Check sheet for the modelled part. Datum: model origin and axes. Units: mm. Face numbers are marked on the shaded views. A direction names the side the tool comes from. Round coordinates to 2 decimals unless told otherwise and drop trailing zeros. Loops run counter-clockwise (first coordinate to the right, second up) from the corner with the lowest first, then second, coordinate; pieces in that order, holes last. Notation, with made-up numbers: (22, -25) -> (79, -25) arc R16 cw to (79, -2) -> close; hole circle Ø7 at (31, 89). An arc over 180 degrees is marked (long way). One line per question, with ' | ' between items.
```python
from build123d import *

# Parameters (mm, degrees)
F0_W     = 50.8
F0_H     = 101.6
F0_W_2   = 101.6
F0_H_2   = 50.8
F1_DEPTH = 38.1
F2_W     = 30.8
F2_H     = 10
F2_W_2   = 10
F2_H_2   = 30.8
F2_W_3   = 30
F2_H_3   = 30
F3_DEPTH = 20
F4_SIZE  = 3
F5_SIZE  = 5


with BuildPart() as f1:
    # F0 (on Top) → F1 (new body)
    with BuildSketch(Plane.XY):
        with BuildLine():
            Line((0, 47.625), (0, 0))
            Line((0, 0), (50.8, 0))
            Line((50.8, 0), (50.8, 50.8))
            Line((50.8, 50.8), (3.175, 50.8))
            ThreePointArc((3.175, 50.8), (2.245064, 48.554936), (0, 47.625))
        make_face()
        with Locations((25.4, -50.8)):
            Rectangle(F0_W, F0_H)
        with Locations((101.6, 25.4)):
            Rectangle(F0_W_2, F0_H_2)
    extrude(amount=F1_DEPTH)

    # F2 (on face) → F3 (cut)
    with BuildSketch(Plane.XY.offset(38.1)):
        with Locations((25.4, -86.6)):
            Rectangle(F2_W, F2_H)
        with Locations((25.4, -61.6)):
            Rectangle(F2_W, F2_H)
        with Locations((25.4, -36.6)):
            Rectangle(F2_W, F2_H)
        with Locations((25.4, -11.6)):
            Rectangle(F2_W, F2_H)
        with Locations((137.4, 25.4)):
            Rectangle(F2_W_2, F2_H_2)
        with Locations((112.4, 25.4)):
            Rectangle(F2_W_2, F2_H_2)
        with Locations((87.4, 25.4)):
            Rectangle(F2_W_2, F2_H_2)
        with Locations((62.4, 25.4)):
            Rectangle(F2_W_2, F2_H_2)
        with Locations((25, 25.8)):
            Rectangle(F2_W_3, F2_H_3)
    extrude(amount=-F3_DEPTH, mode=Mode.SUBTRACT)

    # F4
    f4_edges = [f1.edges().sort_by_distance(p)[0] for p in [
        (10, -6.6, 28.1),
        (10, 40.8, 28.1),
        (10, -31.6, 28.1),
        (10, -56.6, 28.1),
        (10, -81.6, 28.1),
        (10, -91.6, 28.1),
        (40.8, -81.6, 28.1),
        (40.8, -91.6, 28.1),
        (40.8, -66.6, 28.1),
        (40.8, -56.6, 28.1),
        (10, -66.6, 28.1),
        (10, -41.6, 28.1),
        (40.8, -31.6, 28.1),
        (40.8, -41.6, 28.1),
        (10, -16.6, 28.1),
        (40.8, -16.6, 28.1),
        (40.8, -6.6, 28.1),
        (10, 10.8, 28.1),
        (40, 40.8, 28.1),
        (40, 10.8, 28.1),
        (57.4, 40.8, 28.1),
        (57.4, 10, 28.1),
        (67.4, 10, 28.1),
        (67.4, 40.8, 28.1),
        (82.4, 40.8, 28.1),
        (82.4, 10, 28.1),
        (92.4, 40.8, 28.1),
        (92.4, 10, 28.1),
        (107.4, 10, 28.1),
        (117.4, 10, 28.1),
        (117.4, 40.8, 28.1),
        (107.4, 40.8, 28.1),
        (132.4, 10, 28.1),
        (142.4, 10, 28.1),
        (142.4, 40.8, 28.1),
        (132.4, 40.8, 28.1),
    ]]
    chamfer(f4_edges, length=F4_SIZE)

    # F5
    f5_edges = [f1.edges().sort_by_distance(p)[0] for p in [
        (0, -101.6, 19.05),
        (50.8, -101.6, 19.05),
        (152.4, 0, 19.05),
        (152.4, 50.8, 19.05),
    ]]
    chamfer(f5_edges, length=F5_SIZE)


solid = f1.part
```
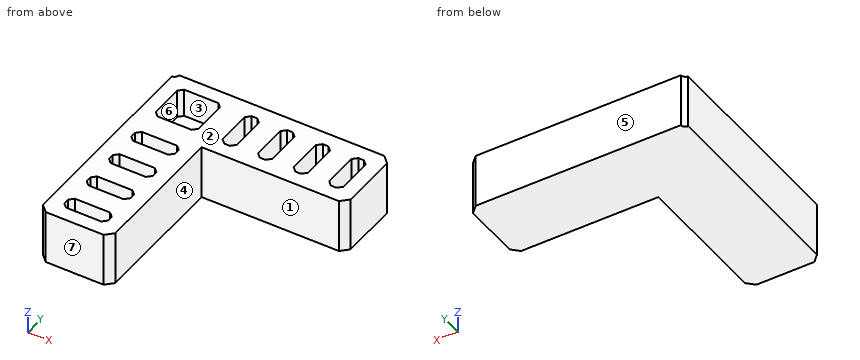
(1) Go/stop test with flat-tipped pins: pin 1 (3 mm diameter, centred on y = -61.5, z = 28.5, fed in from +X); pin 2 (1.5 mm diameter, centred on x = 50, z = 24, fed in from -Y); pin 3 (6 mm diameter, centred on x = 65.5, z = 14.5, fed in from -Y). Record where each tip stops, or that it passes through.
Answer:
pin 1: stops at x = 50.8 | pin 2: stops at y = -98.15 | pin 3: stops at y = 0
(2) Sectioned sample at A-A, the plane z = 9. Record the cut outline in (x, y) (3 decimals).
Answer:
outline: (0, -96.6) -> (5, -101.6) -> (45.8, -101.6) -> (50.8, -96.6) -> (50.8, 0) -> (147.4, 0) -> (152.4, 5) -> (152.4, 45.8) -> (147.4, 50.8) -> (3.175, 50.8) arc R3.175 cw to (0, 47.625) -> close
(3) Mould release check, pull along Y, two halves, no side actions. Record for the marked faces 4, 5, 6 and 7: +Y half, -Y half, draft (parallel to the pull), parting line (faces both ways), or undercut.
Answer:
face 4: draft | face 5: +Y half | face 6: undercut | face 7: -Y half
(4) Sectioned sample at C-C, the plane y = 16.5. Record the cut outline in (x, z), and give its area (3 significant figures).
Answer:
outline: (0, 0) -> (152.4, 0) -> (152.4, 38.1) -> (142.4, 38.1) -> (142.4, 18.1) -> (132.4, 18.1) -> (132.4, 38.1) -> (117.4, 38.1) -> (117.4, 18.1) -> (107.4, 18.1) -> (107.4, 38.1) -> (92.4, 38.1) -> (92.4, 18.1) -> (82.4, 18.1) -> (82.4, 38.1) -> (67.4, 38.1) -> (67.4, 18.1) -> (57.4, 18.1) -> (57.4, 38.1) -> (40, 38.1) -> (40, 18.1) -> (10, 18.1) -> (10, 38.1) -> (0, 38.1) -> close | area: 4,410 mm2
(5) Set-up check for the marked faces 1, 2 and 3: record each of +Z, -Z, +X, -X, +Y, -Y from which the full face is reachable in a straight line by a thin tool's end or side.
Answer:
face 1: +Z, -Z, +X, -Y | face 2: +Z, +X, -X, +Y, -Y | face 3: +Z
(6) Sectioned sample at D-D, the plane z = 26. Count the separate pieces of the cut face and the enclosed holes in it, and give its area (3 significant figures).
Answer:
separate pieces: 1 | enclosed holes: 9 | area: 9,640 mm2
(7) Scan lines: probe 1 along Y at (x, z) = (17, 22.5); probe 2 along X at (y, z) = (35.5, 35); probe 3 along Y at (x, z) = (99, 11). Record each from-to range of solid material in increasing order.
Answer:
probe 1: y = -101.6 to -91.6, -81.6 to -66.6, -56.6 to -41.6, -31.6 to -16.6, -6.6 to 10.8, 40.8 to 50.8 | probe 2: x = 0 to 10, 40 to 57.4, 67.4 to 82.4, 92.4 to 107.4, 117.4 to 132.4, 142.4 to 152.4 | probe 3: y = 0 to 50.8
(8) Sectioned sample at B-B, the plane x = 34. Record the cut outline in (y, z).
Answer:
outline: (-101.6, 0) -> (50.8, 0) -> (50.8, 38.1) -> (40.8, 38.1) -> (40.8, 18.1) -> (10.8, 18.1) -> (10.8, 38.1) -> (-6.6, 38.1) -> (-6.6, 18.1) -> (-16.6, 18.1) -> (-16.6, 38.1) -> (-31.6, 38.1) -> (-31.6, 18.1) -> (-41.6, 18.1) -> (-41.6, 38.1) -> (-56.6, 38.1) -> (-56.6, 18.1) -> (-66.6, 18.1) -> (-66.6, 38.1) -> (-81.6, 38.1) -> (-81.6, 18.1) -> (-91.6, 18.1) -> (-91.6, 38.1) -> (-101.6, 38.1) -> close
